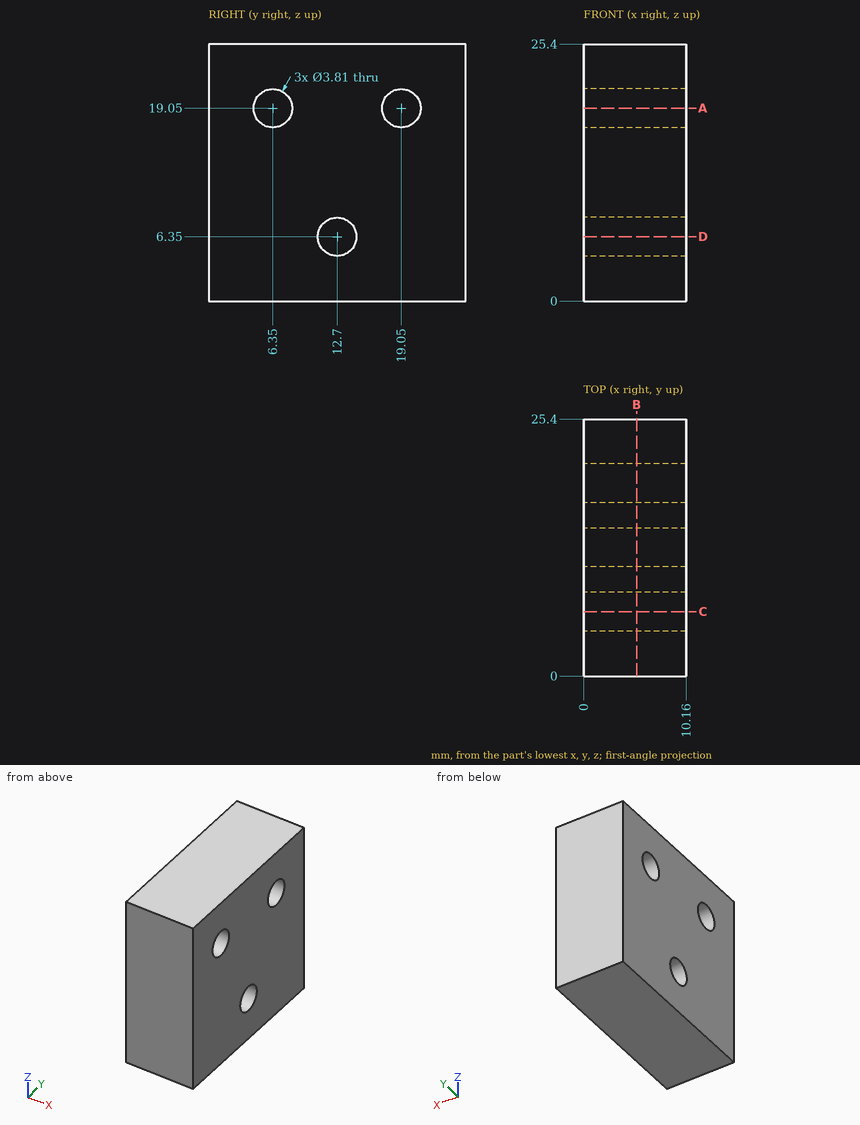
Geometry: see drawing. Coordinates: mm, zero at the bounding-box minimum. Give positions to 0.01 mm unless a question says otherwise; leave off trailing zeros. Write each loop counter-clockwise with the first axis right and the second up, starting at its lowest first coordinate (ties: lowest second). Pieces come first, ordered by that corner, then holes. Notation, with made-up numbers: M -29.5,30.5 L -4.5,30.5 A11 ccw -4.5,42.5 Z; hole C -6,69 d7. An arc over 180 degrees is marked long. Answer as a JSON object with one key per item and string values.
Q1. Cut plane C-C, the plane y = 6.35. Return the cut outline in (x, z) (3 decimals), then the cut area to 3 significant figures.
Geometry check:
{"outline": "M 0,0 L 10.16,0 L 10.16,17.145 L 0,17.145 Z; M 0,20.955 L 10.16,20.955 L 10.16,25.4 L 0,25.4 Z", "area": "219 mm^2"}
Q2. Contact query for flat-ended pins moving along their axis: P1, Ø4, axis at x = 6, z = 20, coming from the -Y side; P2, Ø3, axis at y = 12.7, z = 6.35, coming from the -X side. Output: stop coordinate, or through.
Geometry check:
{"P1": "stops at y = 0", "P2": "passes through"}
Q3. Cut plane B-B, the plane x = 5.25. Return the cut outline in (y, z) (3 decimals), then the cut area to 3 significant figures.
Geometry check:
{"outline": "M 0,0 L 25.4,0 L 25.4,25.4 L 0,25.4 Z; hole C 6.35,19.05 d3.81; hole C 12.7,6.35 d3.81; hole C 19.05,19.05 d3.81", "area": "611 mm^2"}
Q4. Ray query, line 1 along Y through (x, z) = (3.5, 19.05) (3 decimals); line 2 along Y through (x, z) = (7, 6.35) (3 decimals); line 3 along Z through (x, y) = (7.5, 19.05) (3 decimals). Return the intervals inside material, ascending.
Geometry check:
{"line 1": "y = 0 to 4.445, 8.255 to 17.145, 20.955 to 25.4", "line 2": "y = 0 to 10.795, 14.605 to 25.4", "line 3": "z = 0 to 17.145, 20.955 to 25.4"}
Q5. Cut plane A-A, the plane z = 19.05. Return the cut outline in (x, y) (3 decimals).
Geometry check:
{"outline": "M 0,0 L 10.16,0 L 10.16,4.445 L 0,4.445 Z; M 0,8.255 L 10.16,8.255 L 10.16,17.145 L 0,17.145 Z; M 0,20.955 L 10.16,20.955 L 10.16,25.4 L 0,25.4 Z"}
Q6. Cut plane D-D, the plane z = 6.35. Return the cut outline in (x, y) (3 decimals), then the cut area to 3 significant figures.
Geometry check:
{"outline": "M 0,0 L 10.16,0 L 10.16,10.795 L 0,10.795 Z; M 0,14.605 L 10.16,14.605 L 10.16,25.4 L 0,25.4 Z", "area": "219 mm^2"}
